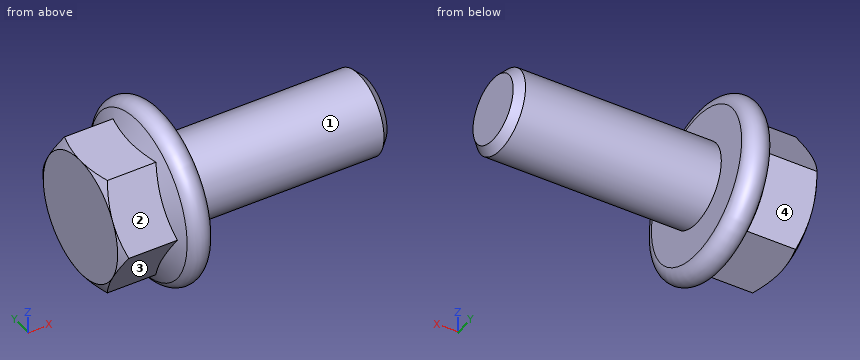
Autodesk Inventor part; units mm, degrees
ref_plane "Work Plane1" through (10.95, 0, 0) normal (0, 0, -1) x (1, 0, 0)
ref_plane "YZ Plane" through (0, 0, 0) normal (1, 0, 0) x (0, 1, 0)
ref_plane "XZ Plane" through (0, 0, 0) normal (0, 1, 0) x (-1, 0, 0)
sketch "Sketch1" plane through (0, 0, 0) normal (0, 0, 1) x (1, 0, 0)
  line L0 (-5.8293, 0) -> (-5.8293, 8.2218)
  line L1 (0, 11.557) -> (0, 6.35)
  line L2 (5.1308, 6.35) -> (31.75, 6.35)
  line L3 (31.75, 6.35) -> (31.75, 0)
  line L4 (31.75, 0) -> (-5.8293, 0)
  arc A0 (0, 11.557) -> (-3.8736, 12.4158) centre (-2.032, 11.557) ccw
  line L5 (0, -2.794) -> (0, 16.7643)
  line L6 (-13.3452, 0) -> (39.2659, 0)
  line L7 (0, 6.35) -> (0.0001, 6.35)
  line L8 (0.0001, 6.35) -> (0.0001, 6.35)
  line L9 (0.0001, 6.35) -> (2.2098, 6.35)
  line L10 (2.2098, 6.35) -> (5.1308, 6.35)
  line L11 (-5.8293, 8.2218) -> (-3.8736, 12.4158)
  line L12 (0.0001, 6.35) -> (5.1308, 6.35) construction
  line L13 (5.1308, 6.35) -> (5.1308, 0) construction
  dimension "d0" = 2.032
  dimension "d1" = 31.75
  dimension "d2" = 26.6192
  dimension "d3" = 27.178
  dimension "d4" = 12.7
  dimension "d5" = 5.8293
  dimension "d15" = 12.7
  dimension "d16" = 12.7
  dimension "d17" = 0.0001
  dimension "d18" = 2.921
  dimension "d19" = 25
revolve "Body" add sketch "Sketch1" angle 360 about axis through (31.75, 0, 0) along (-1, 0, 0)
sketch "Sketch2" plane through (0, 0, 0) normal (1, 0, 0) x (0, 0, -1)
  line L0 (9.525, 5.4993) -> (9.525, -5.4993)
  line L1 (9.525, -5.4993) -> (0, -10.9985)
  line L2 (0, -10.9985) -> (-9.525, -5.4993)
  line L3 (-9.525, -5.4993) -> (-9.525, 5.4993)
  line L4 (-9.525, 5.4993) -> (0, 10.9985)
  line L5 (0, 10.9985) -> (9.525, 5.4993)
  point P0 (0, 0)
  point P1 (0, 0)
  dimension "d23" = 19.05
extrude "Head" add sketch "Sketch2" against normal blind 12.954
sketch "Sketch3" plane through (0, 0, 0) normal (0, 0, 1) x (1, 0, 0)
  line L0 (-12.954, 9.525) -> (-12.954, 10.9985)
  line L1 (-12.954, 10.9985) -> (-12.1033, 10.9985)
  line L2 (-12.1033, 10.9985) -> (-12.954, 9.525)
  line L3 (-14.6379, 0) -> (-2.8506, 0)
  line L4 (-12.954, 10.9985) -> (-12.954, 5.4993)
  line L5 (-4.5345, 10.9985) -> (-12.954, 10.9985)
  point P0 (-12.954, 5.4993)
  dimension "d8" = 30
  dimension "d22" = 19.05
revolve "Chamfer1" cut sketch "Sketch3" angle 360 about axis through (-10, 0, 0) along (1, 0, 0)
thread "Thread"
chamfer "Chamfer2" distance 1.1986 distance2 1.1986 1 edges at (31.75, -6.35, 0) measured on face at (31.75, 0.2551, 2.1012)
ref_plane "Work Plane1" through (10.95, 0, 0) normal (0, 0, -1) x (1, 0, 0)
equation "\"d0\" = PHH"
equation "\"d1\" = NLG"
equation "\"d2\" = GEL"
equation "\"d3\" = LADI"
equation "\"d4\" = GD"
equation "\"d5\" = 0.45 * KOH"
equation "\"d15\" = SD2"
equation "\"d16\" = BDM"
equation "\"d18\" = GAL"
equation "\"d19\" = KEWI"
equation "\"d23\" = SW"
equation "\"d6\" = KOH"
equation "\"d8\" = ANG1"
equation "\"d22\" = SW0"
equation "\"d10\" = GEL"
equation "\"d13\" = -0.5 * SPD + 0.5 * GD"
equation "\"d14\" = GUL"
equation "\"NLG\" = 31.75"
equation "\"GD\" = NND"
equation "\"BDM\" = NND"
equation "\"KOH\" = 12.954"
equation "\"GEL\" = 26.6192"
equation "\"LADI\" = 27.178"
equation "\"SW\" = 19.05"
equation "\"PHH\" = 2.032"
equation "\"SW0\" = SW"
equation "\"SPD\" = 10.30283"
equation "\"SD2\" = NND"
equation "\"SD\" = 0"
equation "\"ANG1\" = 30deg"
equation "\"KEWI\" = 25deg"
equation "\"GAL\" = 2.921"
equation "\"GUL\" = 1.19859"
equation "\"THREADDIA\" = 12.7"
equation "\"SDH\" = SW"
equation "\"TOA\" = 30deg"
equation "\"NND\" = 12.7"
equation "\"E0\" = 1.155 * SW"
equation "\"GD1\" = 10.30283"
properties part number "IFI 111 - 1/2-13 UNC x 1,25" material "Steel, Mild"
CAD build for the part. Positions are in the model's coordinates, mm. Face numbers are marked on the shaded views. A direction names the side the tool comes from. Round coordinates to 2 decimals unless told otherwise and drop trailing zeros. Loops run counter-clockwise (first coordinate to the right, second up) from the corner with the lowest first, then second, coordinate; pieces in that order, holes last. Notation, with made-up numbers: M -31.5,19 L 5.5,19 A21 cw 5.5,26 Z; hole C 77.5,-8.5 d3. An arc over 180 degrees is marked long. One line per question, with ' | ' between items. Start each with the question number.
Item 1: Pin check, flat tips, straight feed: pin 1 Ø1.5 at (x, z) = (18, 1.5) entering from -Y; pin 2 Ø6.5 at (x, y) = (-10.5, -0.5) entering from +Z (3 decimals); pin 3 Ø4 at (x, y) = (16, 6) entering from -Z. Stop position of each tip, or through.
Item 2: Wall check: line 1 (X direction, y = -2, z = -9); line 2 (Y direction, x = -9, z = 0); line 3 (X direction, y = 1.5, z = 10.25). Give the ranges that are in metal, low to high.
Item 3: Which spindle directions (+Z, -Z, +X, -X, +Y, -Y) get a long thin tool onto all of the face, cutting with end or side? Do the marked faces 1, 2, 3 and 4. Say none if no direction does.
Item 4: Cut at A-A, the plane x = 14.5. Write the cut outline in (y, z).
Responses:
1) pin 1: stops at y = -6.31 | pin 2: stops at z = 9.525 | pin 3: stops at z = -4.93
2) line 1: x = -12.95 to 0 | line 2: y = -11 to 11 | line 3: x = -4.83 to 0
3) face 1: +X | face 2: +Z, -X, -Y | face 3: -Z, -X, -Y | face 4: -Z, -X, +Y
4) outline: C 0,0 d12.7
